Geometry: final body of the model. Coordinates: model frame, mm. Face numbers are marked on the shaded views. A direction names the side the tool comes from. Give positions to 0.01 mm unless a question says otherwise; leave off trailing zeros. Write each loop counter-clockwise with the first axis right and the second up, starting at its lowest first coordinate (ties: lowest second). Pieces come first, ordered by that corner, then holes. Notation, with made-up numbers: M 27.5,-19 L 37.5,-19 A29 cw 37.5,16 Z; hole C 63,77 d9. An arc over 180 degrees is marked long. Use a Markdown table: item, result. Add a question column.
(1) Cut plane B-B (x = 120). Output: boundary loops of the cut face in (y, z), plus the area to 3 significant figures.
(2) Cut plane C-C (y = 25). Output: boundary loops of the cut face in (x, z).
(3) Reachability of the marked faces 4 and 5 from +Z, -Z, +X, -X, +Y, -Y: full face, straight path, thin tool, end or side. Return the list, or none.
(4) Cut plane D-D (y = 40). Output: boundary loops of the cut face in (x, z), plus the area to 3 significant figures.
(5) Material intervals for L1, parallel to Y at x = 230, z = 2; L2, parallel to Z at x = 19, y = 47.5; L3, parallel to X at y = 30.5, z = 8.75, sorted ascending.
(6) Pin query (flat end, axial travel): pin 1 Ø1.5 at (y, z) = (36.5, 11.5) entering from -X; pin 2 Ø2 at (x, y) = (101, 48) entering from -Z; pin 3 Ø6 at (x, y) = (63.5, 11.5) entering from +Z. Return the tip coordinate at first contact, or that it passes through.
(7) Draft query along Y for the marked faces 1, 2 and 3. Return one class per face: released by +Y, released by -Y, zero draft, split by the parting line, or undercut.
(8) Cut plane A-A (x = 10). Output: boundary loops of the cut face in (y, z), plus the area to 3 significant figures.
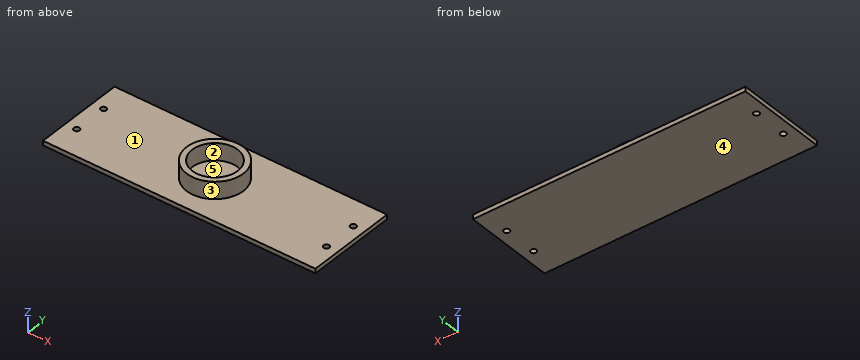
```python
from build123d import *

# Parameters (mm, degrees)
ESQUISSE1_W        = 240
ESQUISSE1_H        = 80
ESQUISSE1_R        = 2.5
BOSS_EXTRU_1_DEPTH = 4
ESQUISSE2_R        = 25
ESQUISSE2_R_2      = 20
BOSS_EXTRU_2_DEPTH = 15


with BuildPart() as part:
    # Esquisse1 → Boss.-Extru.1 (new body)
    with BuildSketch(Plane.XY):
        with Locations((120, 40)):
            Rectangle(ESQUISSE1_W, ESQUISSE1_H)
        with Locations((10, 55)):
            Circle(ESQUISSE1_R, mode=Mode.SUBTRACT)
        with Locations((10, 25)):
            Circle(ESQUISSE1_R, mode=Mode.SUBTRACT)
        with Locations(Location((230, 25, 0), (0, 0, 180))):
            Circle(ESQUISSE1_R, mode=Mode.SUBTRACT)
        with Locations(Location((230, 55, 0), (0, 0, 180))):
            Circle(ESQUISSE1_R, mode=Mode.SUBTRACT)
    extrude(amount=BOSS_EXTRU_1_DEPTH)

    # Esquisse2 → Boss.-Extru.2 (add)
    with BuildSketch(Plane.XY.offset(4)):
        with Locations(Location((120, 40, 0), (0, 0, 180))):
            Circle(ESQUISSE2_R)
        with Locations((120, 40)):
            Circle(ESQUISSE2_R_2, mode=Mode.SUBTRACT)
    extrude(amount=BOSS_EXTRU_2_DEPTH)


solid = part.part
```
Answer list:
| question | item | result |
|---|---|---|
| 1 | outline | M 0,0 L 80,0 L 80,4 L 65,4 L 65,19 L 60,19 L 60,4 L 20,4 L 20,19 L 15,19 L 15,4 L 0,4 Z |
| 1 | area | 470 mm² |
| 2 | outline | M 0,0 L 7.5,0 L 7.5,4 L 0,4 Z; M 12.5,0 L 227.5,0 L 227.5,4 L 140,4 L 140,19 L 133.23,19 L 133.23,4 L 106.77,4 L 106.77,19 L 100,19 L 100,4 L 12.5,4 Z; M 232.5,0 L 240,0 L 240,4 L 232.5,4 Z |
| 3 | face 4 | -Z, +X, -X, +Y, -Y |
| 3 | face 5 | +Z |
| 4 | outline | M 0,0 L 240,0 L 240,4 L 145,4 L 145,19 L 140,19 L 140,4 L 100,4 L 100,19 L 95,19 L 95,4 L 0,4 Z |
| 4 | area | 1,110 mm² |
| 5 | L1 | 0 to 22.5, 27.5 to 52.5, 57.5 to 80 |
| 5 | L2 | 0 to 4 |
| 5 | L3 | 96.88 to 102.4, 137.6 to 143.12 |
| 6 | pin 1 | x = 95.15 |
| 6 | pin 2 | z = 0 |
| 6 | pin 3 | z = 4 |
| 7 | face 1 | zero draft |
| 7 | face 2 | undercut |
| 7 | face 3 | split by the parting line |
| 8 | outline | M 0,0 L 22.5,0 L 22.5,4 L 0,4 Z; M 27.5,0 L 52.5,0 L 52.5,4 L 27.5,4 Z; M 57.5,0 L 80,0 L 80,4 L 57.5,4 Z |
| 8 | area | 280 mm² |
